Geometry: final body of the model. Coordinates: model frame, mm. A direction names the side the tool comes from. Give positions to 0.01 mm unless a question says otherwise; leave off trailing zeros. Order: outer loops, then holes, each group sorted by start corner. A loop starts at its lowest first (then second) coordinate and runs counter-clockwise, first axis right, second up. Notation, with made-up numbers: (74.25, -13) -> (130.25, -13) arc R7 cw to (130.25, -5) -> close; hole circle Ø11 at (88.5, 63.25). An arc over 180 degrees is marked (long way). One line per question, with ' | ' between items.
from build123d import *

# Parameters (mm, degrees)
SKETCH_1_W          = 20
SKETCH_1_H          = 15
SKETCH_1_W_2        = 18
SKETCH_1_H_2        = 13
EXTRUDE_1_DEPTH     = 200
SKETCH_3_R          = 1.6
CUT_EXTRUDE_1_DEPTH = 201.81085628
SKETCH_4_R          = 1.6
CUT_EXTRUDE_2_DEPTH = 202.137390855


with BuildPart() as part:
    # 草图1 → 拉伸-薄壁1 (new body)
    with BuildSketch(Plane(origin=(0, 0, 0), x_dir=(1, 0, 0), z_dir=(0, 1, 0))):
        Rectangle(SKETCH_1_W, SKETCH_1_H)
        Rectangle(SKETCH_1_W_2, SKETCH_1_H_2, mode=Mode.SUBTRACT)
    extrude(amount=EXTRUDE_1_DEPTH)

    # 草图3 → 切除-拉伸1 (cut, through all)
    with BuildSketch(Plane.XY.offset(7.5)):
        with Locations((-5, 153)):
            Circle(SKETCH_3_R)
        with Locations(Location((-5, 143, 0), (0, 0, 180))):
            Circle(SKETCH_3_R)
        with Locations((5, 143)):
            Circle(SKETCH_3_R)
        with Locations(Location((5, 153, 0), (0, 0, 180))):
            Circle(SKETCH_3_R)
    extrude(amount=-CUT_EXTRUDE_1_DEPTH, mode=Mode.SUBTRACT)

    # 草图4 → 切除-拉伸2 (cut, through all)
    with BuildSketch(Plane(origin=(10, 0, 0), x_dir=(0, 0, -1), z_dir=(1, 0, 0))):
        with Locations((-3.75, 5)):
            Circle(SKETCH_4_R)
        with Locations((-3.75, 15)):
            Circle(SKETCH_4_R)
        with Locations((3.75, 5)):
            Circle(SKETCH_4_R)
        with Locations((3.75, 15)):
            Circle(SKETCH_4_R)
        with Locations((3.75, 185)):
            Circle(SKETCH_4_R)
        with Locations((3.75, 195)):
            Circle(SKETCH_4_R)
        with Locations((-3.75, 185)):
            Circle(SKETCH_4_R)
        with Locations((-3.75, 195)):
            Circle(SKETCH_4_R)
    extrude(amount=-CUT_EXTRUDE_2_DEPTH, mode=Mode.SUBTRACT)


solid = part.part
1) Pull-direction query (X, two-part tool) for faces 1 (the cylindrical face through (-4.65, 144.56, -6.99)), 2 (the flat face through (-10, 99, 0)), 3 (the cylindrical face through (9.51, 3.58, -4.49)), 4 (the cylindrical face through (5.35, 154.56, 7.01)); classes: +X half, -X half, draft (parallel to the pull), parting line (faces both ways), or undercut.
Check result:
face 1: undercut | face 2: -X half | face 3: draft | face 4: undercut
2) Section A-A on x = 1.75. Return loops of the section in (y, z), plus the area to 3 significant figures.
Check result:
outline: (0, -7.5) -> (200, -7.5) -> (200, -6.5) -> (0, -6.5) -> close; (0, 6.5) -> (200, 6.5) -> (200, 7.5) -> (0, 7.5) -> close | area: 400 mm^2
3) Section B-B on y = 37. Return loops of the section in (x, z), plus the area to 3 significant figures.
Check result:
outline: (-10, -7.5) -> (10, -7.5) -> (10, 7.5) -> (-10, 7.5) -> close; hole (-9, -6.5) -> (9, -6.5) -> (9, 6.5) -> (-9, 6.5) -> close | area: 66.0 mm^2
4) Contact query for flat-ended pins moving along their axis: pin 1 Ø5 at (x, z) = (-4, 3.5) entering from -Y; pin 2 Ø4 at (y, z) = (195, -3.75) entering from +X. Output: stop coordinate, or through.
Check result:
pin 1: passes through | pin 2: stops at x = 10
5) Set-up query: faces 5 (the flat face through (0, 99, -7.5)), 6 (the flat face through (0, 99, -6.5)). Return all of +Z, -Z, +X, -X, +Y, -Y with unobstructed straight access to the full face (end or side cutting, diameter ignored); none if empty.
Check result:
face 5: -Z, +X, -X, +Y, -Y | face 6: +Y, -Y
6) Material intervals for probe 1 along Y at (x, z) = (9.45, 3.75); probe 2 along Z at (x, y) = (8.25, 186); probe 3 along X at (y, z) = (31, -5.5), sorted ascending. Write a range as from..to.
Check result:
probe 1: y = 0..3.4, 6.6..13.4, 16.6..183.4, 186.6..193.4, 196.6..200 | probe 2: z = -7.5..-6.5, 6.5..7.5 | probe 3: x = -10..-9, 9..10
